Can you work these out from the model? Positions are in its coordinate system, mm. A direction names the side the tool comes from. Round coordinates to 2 decimals unless told otherwise and drop trailing zeros. Order: outer loops, then holes, each group sorted by start corner. A loop starts at its lowest first (then second) coordinate and runs counter-clockwise, first axis right, second up. Notation, with made-up numbers: M 43,-33 L 59,-33 A25 ccw 59,-10 Z; hole C 71.25,-28.75 d9. An arc over 180 degrees is marked long. Answer as a JSON object with one key per item and string values. Group by question number.
```python
from build123d import *

# Parameters (mm, degrees)
SALIENTE_EXTRUIR1_OUTLINE_W   = 70
SALIENTE_EXTRUIR1_OUTLINE_H   = 121
SALIENTE_EXTRUIR1_OUTLINE_W_2 = 21.402751614
SALIENTE_EXTRUIR1_OUTLINE_H_2 = 22.176249264
SALIENTE_EXTRUIR1_DEPTH       = 3
CROQUIS3_W                    = 70
CROQUIS3_H                    = 121
CROQUIS3_W_2                  = 66
CROQUIS3_H_2                  = 117
SALIENTE_EXTRUIR2_DEPTH       = 25
CROQUIS6_R                    = 2
CORTAR_EXTRUIR1_DEPTH         = 10


# Read off the part's stored shape, not the designer's step: Saliente-Extruir1
with BuildPart() as part:
    # Saliente-Extruir1 outline → Saliente-Extruir1 (new body)
    with BuildSketch(Plane.XY):
        Rectangle(SALIENTE_EXTRUIR1_OUTLINE_W, SALIENTE_EXTRUIR1_OUTLINE_H)
        with BuildLine():
            Line((10.665295135, -26.794102385), (18.701771575, -26.794102385))
            ThreePointArc((18.701771575, -26.794102385), (19.408878356, -27.086995604), (19.701771575, -27.794102385))
            Line((19.701771575, -27.794102385), (19.701771575, -35.634526795))
            ThreePointArc((19.701771575, -35.634526795), (19.408878356, -36.341633576), (18.701771575, -36.634526795))
            Line((18.701771575, -36.634526795), (10.665295135, -36.634526795))
            ThreePointArc((10.665295135, -36.634526795), (9.958188354, -36.341633576), (9.665295135, -35.634526795))
            Line((9.665295135, -35.634526795), (9.665295135, -27.794102385))
            ThreePointArc((9.665295135, -27.794102385), (9.958188354, -27.086995604), (10.665295135, -26.794102385))
        make_face(mode=Mode.SUBTRACT)
        with BuildLine():
            Line((10.057242416, -19.858648736), (10.057242416, -12.018224326))
            ThreePointArc((10.057242416, -12.018224326), (10.350135635, -11.311117545), (11.057242416, -11.018224326))
            Line((11.057242416, -11.018224326), (18.701771575, -11.018224326))
            ThreePointArc((18.701771575, -11.018224326), (19.408878356, -11.311117545), (19.701771575, -12.018224326))
            Line((19.701771575, -12.018224326), (19.701771575, -19.858648736))
            ThreePointArc((19.701771575, -19.858648736), (19.408878356, -20.565755517), (18.701771575, -20.858648736))
            Line((18.701771575, -20.858648736), (11.057242416, -20.858648736))
            ThreePointArc((11.057242416, -20.858648736), (10.350135635, -20.565755517), (10.057242416, -19.858648736))
        make_face(mode=Mode.SUBTRACT)
        with Locations((-9.158031826, 28.317647119)):
            Rectangle(SALIENTE_EXTRUIR1_OUTLINE_W_2, SALIENTE_EXTRUIR1_OUTLINE_H_2, mode=Mode.SUBTRACT)
        with BuildLine():
            Line((9.665295135, -1.437126531), (9.665295135, 6.207324239))
            ThreePointArc((9.665295135, 6.207324239), (9.958188354, 6.91443102), (10.665295135, 7.207324239))
            Line((10.665295135, 7.207324239), (18.701771575, 7.207324239))
            ThreePointArc((18.701771575, 7.207324239), (19.408878356, 6.91443102), (19.701771575, 6.207324239))
            Line((19.701771575, 6.207324239), (19.701771575, -1.437126531))
            ThreePointArc((19.701771575, -1.437126531), (19.408878356, -2.144233312), (18.701771575, -2.437126531))
            Line((18.701771575, -2.437126531), (10.665295135, -2.437126531))
            ThreePointArc((10.665295135, -2.437126531), (9.958188354, -2.144233312), (9.665295135, -1.437126531))
        make_face(mode=Mode.SUBTRACT)
        with BuildLine():
            Line((9.861268776, 15.612580192), (9.861268776, 23.453004601))
            ThreePointArc((9.861268776, 23.453004601), (10.154161995, 24.160111382), (10.861268776, 24.453004601))
            Line((10.861268776, 24.453004601), (18.505797934, 24.453004601))
            ThreePointArc((18.505797934, 24.453004601), (19.212904715, 24.160111382), (19.505797934, 23.453004601))
            Line((19.505797934, 23.453004601), (19.505797934, 15.612580192))
            ThreePointArc((19.505797934, 15.612580192), (19.212904715, 14.905473411), (18.505797934, 14.612580192))
            Line((18.505797934, 14.612580192), (10.861268776, 14.612580192))
            ThreePointArc((10.861268776, 14.612580192), (10.154161994, 14.90547341), (9.861268776, 15.612580192))
        make_face(mode=Mode.SUBTRACT)
    extrude(amount=SALIENTE_EXTRUIR1_DEPTH)

    # Croquis3 → Saliente-Extruir2 (add)
    with BuildSketch(Plane(origin=(0, 0, 0), x_dir=(-1, 0, 0), z_dir=(0, 0, -1))):
        Rectangle(CROQUIS3_W, CROQUIS3_H)
        Rectangle(CROQUIS3_W_2, CROQUIS3_H_2, mode=Mode.SUBTRACT)
    extrude(amount=SALIENTE_EXTRUIR2_DEPTH)

    # Croquis6 → Cortar-Extruir1 (cut)
    with BuildSketch(Plane.XY.offset(3)):
        with Locations((-27, 52.5)):
            Circle(CROQUIS6_R)
        with Locations(Location((-27, -52.5, 0), (0, 0, 180))):
            Circle(CROQUIS6_R)
        with Locations((27, -52.5)):
            Circle(CROQUIS6_R)
        with Locations(Location((27, 52.5, 0), (0, 0, 180))):
            Circle(CROQUIS6_R)
    extrude(amount=-CORTAR_EXTRUIR1_DEPTH, mode=Mode.SUBTRACT)


solid = part.part
```
1) We'd pull the mould along Y, two halves only. Please class faces 1 (the face through (-35, -1, -11)), 2 (the face through (0, 58.5, -12)): +Y half, -Y half, draft (parallel to the pull), parting line (faces both ways), or undercut.
2) If we section it at B-B on x = -3: Write out the boundary of the cut face in (y, z).
3) If we section it at D-D on y = 52.5: Write out the boundary of the cut face in (x, z), plus the area to 3 significant figures.
4) If we section it at C-C on z = -20: Write out the boundary of the cut face in (x, y), plus the area to 3 significant figures.
5) For pin 1 (4 mm diameter, centred on x = -5, y = 18.5, fed in from -Z), with a flat end and sliding along its axis, tell me the tip position at first contact or that it passes through.
6) I need wall thicknesses on line 1 along Y through (x, z) = (12.5, 0.5); line 2 along Y through (x, z) = (27, 0.95); line 3 along X through (y, z) = (7, -6.25). Which ranges of each line are inside material? Lowest first, please.
7) Which directions (+Z, -Z, +X, -X, +Y, -Y) give clear straight access to the entire face, cutting with the end or side of a thin tool? Please do faces 3 (the face through (15, 24.453, 1)), 4 (the face through (0, 1, 3)), 5 (the face through (-33, -1, -12)).
8) If we section it at A-A on y = 2: Write out the boundary of the cut face in (x, z), plus the area to 3 significant figures.
Findings:
{
 "1": {"face 1": "draft", "face 2": "undercut"},
 "2": {"outline": "M -60.5,-25 L -58.5,-25 L -58.5,0 L 17.23,0 L 17.23,3 L -60.5,3 Z; M 39.41,0 L 58.5,0 L 58.5,-25 L 60.5,-25 L 60.5,3 L 39.41,3 Z"},
 "3": {"outline": "M -35,-25 L -33,-25 L -33,0 L -29,0 L -29,3 L -35,3 Z; M -25,0 L 25,0 L 25,3 L -25,3 Z; M 29,0 L 33,0 L 33,-25 L 35,-25 L 35,3 L 29,3 Z", "area": "286 mm^2"},
 "4": {"outline": "M -35,-60.5 L 35,-60.5 L 35,60.5 L -35,60.5 Z; hole M -33,-58.5 L 33,-58.5 L 33,58.5 L -33,58.5 Z", "area": "748 mm^2"},
 "5": {"pin 1": "stops at z = 0"},
 "6": {"line 1": "y = -60.5 to -36.63, -26.79 to -20.86, -11.02 to -2.44, 7.21 to 14.61, 24.45 to 60.5", "line 2": "y = -60.5 to -54.5, -50.5 to 50.5, 54.5 to 60.5", "line 3": "x = -35 to -33, 33 to 35"},
 "7": {"face 3": "+Z, -Z", "face 4": "+Z, +X, -X, +Y, -Y", "face 5": "-Z"},
 "8": {"outline": "M -35,-25 L -33,-25 L -33,0 L 9.67,0 L 9.67,3 L -35,3 Z; M 19.7,0 L 33,0 L 33,-25 L 35,-25 L 35,3 L 19.7,3 Z", "area": "280 mm^2"}
}
